from build123d import *

# Parameters (mm, degrees)
F0_W      = 76.2
F0_H      = 76.2
F1_DEPTH  = 76.2
F2_W      = 25.4
F2_H      = 25.4
F3_DEPTH  = 6.35
F4_R      = 12.7
F5_DEPTH  = 12.7
F7_D      = 25.4
F9_DEPTH  = 25.4
F11_DEPTH = 25.4
F12_DEPTH = 127


with BuildPart() as f1:
    # F0 (on Front) → F1 (new body)
    with BuildSketch(Plane.XZ):
        with Locations((-36.9649222121, 39.7534392561)):
            Rectangle(F0_W, F0_H)
    extrude(amount=F1_DEPTH)

    # F2 (on face) → F3 (join)
    with BuildSketch(Plane.XZ.offset(76.2)):
        with Locations((-44.3486804143, 39.7534392561)):
            Rectangle(F2_W, F2_H)
    extrude(amount=F3_DEPTH)

    # F4 (on face) → F5 (join)
    with BuildSketch(Plane.YZ.offset(1.1350777879)):
        with Locations((-50.8, 52.4534392561)):
            Circle(F4_R)
    extrude(amount=F5_DEPTH)

    # F7 (through all)
    with Locations(Plane.XY.offset(77.8534392561)):
        with Locations((-36.9649222121, -38.1)):
            Hole(F7_D / 2)

    # F8 (on face) → F9 (join)
    with BuildSketch(Plane(origin=(-75.0649222121, 0, 0), x_dir=(0, -1, 0), z_dir=(-1, 0, 0))):
        Polygon((28.7754268733, 47.5637023159), (52.9997243198, 55.2019883295), (34.2726258674, 72.3617023001), align=None)
    extrude(amount=F9_DEPTH)

    # F10 (on face) → F11 (join)
    with BuildSketch(Plane(origin=(0, 0, 0), x_dir=(-1, 0, 0), z_dir=(0, 1, 0))):
        Polygon((48.0731389709, 54.716393042), (47.494721, 47.9351072785), (43.6031534613, 42.3515505225), (37.4411787343, 39.4618322976), (30.6598929708, 40.0402502686), (25.0763362148, 43.9318178073), (22.1866179899, 50.0937925343), (22.7650359609, 56.8750782978), (26.2971690254, 61.9429244137), (4.4938835457, 65.529052283), (14.595719446, 77.8534392561), (-1.1350777879, 77.8534392561), (-1.1350777879, 1.6534392561), (75.0649222121, 1.6534392561), (75.0649222121, 77.8534392561), (23.3556207336, 77.8534392561), (28.7842644927, 63.4564224548), (32.8185782266, 65.3483532786), (39.5998639901, 64.7699353076), (45.1834207461, 60.878367769), align=None)
    extrude(amount=F11_DEPTH)

    # F12 (add): a face of the model
    f12_faces = [f1.faces().sort_by_distance(p)[0] for p in [
        (-29.6209638301, 0, 57.8915936643),
    ]]
    extrude(f12_faces, amount=F12_DEPTH)


solid = f1.part
Source: CAD feature listing. Evaluate the final solid. Frame: model axes, mm. A direction names the side the tool comes from. Coordinates: 2 decimals unless noted, no trailing zeros. Order: outer loops, then holes, each group sorted by start corner. A loop starts at its lowest first (then second) coordinate and runs counter-clockwise, first axis right, second up.
Item 1: First-contact query: P1, Ø5, axis at y = -34.5, z = 57, coming from the +X side; P2, Ø23, axis at x = -36.96, y = -38.1, coming from the -Z side; P3, Ø2, axis at y = -58.5, z = 70, coming from the -X side; P4, Ø5, axis at y = -79, z = 40.5, coming from the +X side. Flat tips, straight axial feed; report the tip coordinate or a pass-through.
Output values:
P1: stops at x = 1.14
P2: passes through
P3: stops at x = -75.06
P4: stops at x = -31.65
Item 2: Cut plane C-C (y = -22.5). Return loops of the section in (x, z).
Output values:
outline: (-75.06, 1.65) - (1.14, 1.65) - (1.14, 77.85) - (-75.06, 77.85) - close
Item 3: Material intervals for line 1 (X direction, y = -38, z = 61); line 2 (X direction, y = -53, z = 38.5); line 3 (Y direction, x = -69, z = 36), sorted ascending.
Output values:
line 1: x = -100.46 to -49.66, -24.27 to 1.14
line 2: x = -75.06 to 1.14
line 3: y = -76.2 to 25.4
Item 4: Cut plane A-A (z = 31). Return loops of the section in (x, y), plus the area to 3 significant figures.
Output values:
outline: (-75.06, -76.2) - (-57.05, -76.2) - (-57.05, -82.55) - (-31.65, -82.55) - (-31.65, -76.2) - (1.14, -76.2) - (1.14, 25.4) - (-75.06, 25.4) - close; hole circle Ø25.4 at (-36.96, -38.1)
area: 7,400 mm2
Item 5: Cut plane B-B (y = 31.5). Return loops of the section in (x, z), plus the area to 3 significant figures.
Output values:
outline: (-48.07, 54.72) - (-47.49, 47.94) - (-43.6, 42.35) - (-37.44, 39.46) - (-30.66, 40.04) - (-25.08, 43.93) - (-22.19, 50.09) - (-22.77, 56.88) - (-26.3, 61.94) - (-4.49, 65.53) - (-14.6, 77.85) - (-23.36, 77.85) - (-28.78, 63.46) - (-32.82, 65.35) - (-39.6, 64.77) - (-45.18, 60.88) - close
area: 762 mm2
Item 6: Set-up query: faces 1 (the face through (-40.57, 75.49, 40.93)), 2 (the face through (-9.47, 75.49, 71.6)), 3 (the face through (-87.59, -43.77, 63.66)). Return all of +Z, -Z, +X, -X, +Y, -Y with unobstructed straight access to the full face (end or side cutting, diameter ignored); none if empty.
Output values:
face 1: -Z, -X, +Y
face 2: +Z, +X, +Y
face 3: +Z, -X, -Y
Item 7: Pull-direction query (Z, two-part tool) for faces 4 (the face through (7.396, -52.453, 65.045)), 5 (the face through (-24.506, 75.489, 59.374)), 6 (the face through (-22.472, 75.489, 53.437)), 7 (the face through (-42.353, 75.489, 62.851)); classes: pulls with the +Z half, pulls with the -Z half, needs draft (parallel to the pull), parting line crosses it, or undercut.
Output values:
face 4: parting line crosses it
face 5: undercut
face 6: undercut
face 7: pulls with the +Z half
